Check sheet for the modelled part. Datum: model origin and axes. Units: mm. Face numbers are marked on the shaded views. A direction names the side the tool comes from. Round coordinates to 2 decimals unless told otherwise and drop trailing zeros. Write each loop counter-clockwise with the first axis right and the second up, starting at its lowest first coordinate (ties: lowest second). Pieces come first, ordered by that corner, then holes. Notation, with made-up numbers: M 60.25,-20 L 96.25,-20 A26 cw 96.25,9 Z; hole C 8,33 d2. An arc over 180 degrees is marked long. Answer in a Markdown table with one row per item.
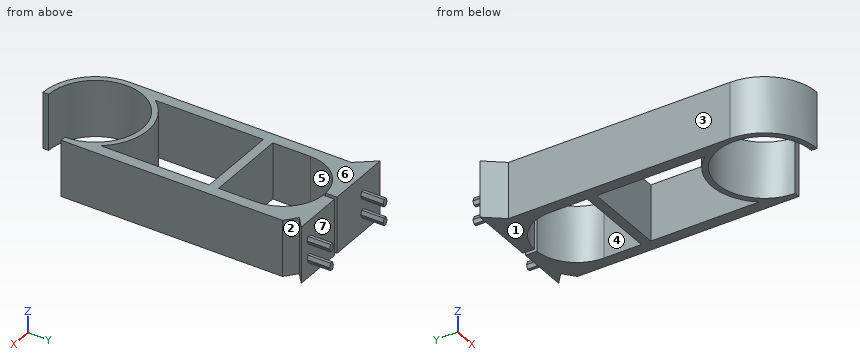
```python
from build123d import *

# Parameters (mm, degrees)
PAD_DEPTH    = 30
PAD001_DEPTH = 12


with BuildPart() as part:
    # Sketch → Pad (new body)
    with BuildSketch(Plane.XY):
        with BuildLine():
            ThreePointArc((25, 0), (-17.67767, 17.67767), (0, -25))
            Line((0, -25), (0, -28))
            ThreePointArc((-28, 1.4e-05), (-19.798995, -19.798985), (0, -28))
            Line((-28, 100.000014), (-28, 1.4e-05))
            Line((-28, 118.000014), (-28, 100.000014))
            Line((-36, 128), (-28, 118.000014))
            Line((-36, 128), (-1, 128))
            Line((-1, 128), (-1, 121.977261))
            ThreePointArc((-1, 121.977261), (-15.905969, 115.198689), (-22, 100.000014))
            Line((-22, 100.000014), (-22, 80))
            Line((-22, 80), (22, 80))
            Line((22, 100), (22, 80))
            ThreePointArc((22, 100), (15.905974, 115.198684), (1, 121.977261))
            Line((1, 128), (1, 121.977261))
            Line((1, 128), (28, 128))
            Line((28, 128), (22, 123))
            Line((22, 123), (28, 118))
            Line((28, 118), (28, 100))
            Line((28, 100), (28, 0))
            Line((25, 0), (28, 0))
        make_face()
        with BuildLine():
            ThreePointArc((22, 17.320508), (0, 28), (-22, 17.320508))
            Line((-22, 75), (-22, 17.320508))
            Line((-22, 75), (22, 75))
            Line((22, 75), (22, 17.320508))
        make_face(mode=Mode.SUBTRACT)
    extrude(amount=PAD_DEPTH)

    # Sketch001 (on Face13 of Pad) → Pad001 (join)
    with BuildSketch(Plane(origin=(0, 128, 0), x_dir=(-1, 0, 0), z_dir=(0, 1, 0))):
        Polygon((-22.5, 12), (-23.3, 10), (-22.5, 8), (-21, 8), (-20.2, 10), (-21, 12), align=None)
        Polygon((-22.5, 22), (-23.3, 20), (-22.5, 18), (-21, 18), (-20.2, 20), (-21, 22), align=None)
        Polygon((21, 12), (20.2, 10), (21, 8), (22.5, 8), (23.3, 10), (22.5, 12), align=None)
        Polygon((21, 22), (20.2, 20), (21, 18), (22.5, 18), (23.3, 20), (22.5, 22), align=None)
    extrude(amount=PAD001_DEPTH)


solid = part.part
```
1. Section check B-B, the plane z = 2.5. Record the cut outline in (x, y).
Found:
| item | result |
|---|---|
| outline | M -36,128 L -28,118 L -28,0 A28 ccw 0,-28 L 0,-25 A25 cw long 25,0 L 28,0 L 28,118 L 22,123 L 28,128 L 1,128 L 1,121.98 A22 cw 22,100 L 22,80 L -22,80 L -22,100 A22 cw -1,121.98 L -1,128 Z; hole M -22,17.32 A28 cw 22,17.32 L 22,75 L -22,75 Z |
2. Draft check along Y on the marked faces 5, 6 and 7. Enter one of: +Y half, -Y half, draft (parallel to the pull), parting line (faces both ways), or undercut.
Found:
| item | result |
|---|---|
| face 5 | undercut |
| face 6 | draft |
| face 7 | +Y half |
3. Section check D-D, the plane x = 13.5. Record the cut outline in (y, z), and give its area (3 significant figures).
Found:
| item | result |
|---|---|
| outline | M 21.04,0 L 24.53,0 L 24.53,30 L 21.04,30 Z; M 75,0 L 80,0 L 80,30 L 75,30 Z; M 117.37,0 L 128,0 L 128,30 L 117.37,30 Z |
| area | 574 mm2 |
4. Access from +Z, -Z, +X, -X, +Y, -Y to the whole of each face (thin tool, end or side, straight path). Record for the marked faces 1, 2, 3 and 4.
Found:
| item | result |
|---|---|
| face 1 | -Z, +X, -X, +Y, -Y |
| face 2 | +Z, -Z, +X |
| face 3 | +Z, -Z, -X, -Y |
| face 4 | +Z, -Z |
5. Scan lines: L1, parallel to X at y = 32.5, z = 24.25; L2, parallel to Y at x = 7, z = 9.5; L3, parallel to Y at x = -18.5, z = 8.25. Record each from-to range of solid material in increasing order.
Found:
| item | result |
|---|---|
| L1 | x = -28 to -22, 22 to 28 |
| L2 | y = 24 to 27.11, 75 to 80, 120.86 to 128 |
| L3 | y = -21.02 to -16.82, 16.82 to 21.02, 75 to 80, 111.91 to 128 |
6. Section check C-C, the plane x = -10. Record the cut outline in (y, z).
Found:
| item | result |
|---|---|
| outline | M -26.15,0 L -22.91,0 L -22.91,30 L -26.15,30 Z; M 22.91,0 L 26.15,0 L 26.15,30 L 22.91,30 Z; M 75,0 L 80,0 L 80,30 L 75,30 Z; M 119.6,0 L 128,0 L 128,30 L 119.6,30 Z |
7. Section check A-A, the plane y = 67. Record the cut outline in (x, z), and give its area (3 significant figures).
Found:
| item | result |
|---|---|
| outline | M -28,0 L -22,0 L -22,30 L -28,30 Z; M 22,0 L 28,0 L 28,30 L 22,30 Z |
| area | 360 mm2 |
8. Go/stop test with flat-tipped pins: pin 1 (1.6 mm diameter, centred on x = 22, y = 134, fed in from +Z); pin 2 (5 mm diameter, centred on x = -29, y = -11, fed in from +Z); pin 3 (1 mm diameter, centred on y = -0.5, z = 24.5, fed in from -X); pin 4 (10 mm diameter, centred on x = -6, z = 19.5, fed in from -Y). Record where each tip stops, or that it passes through.
Found:
| item | result |
|---|---|
| pin 1 | stops at z = 22 |
| pin 2 | passes through |
| pin 3 | stops at x = -28 |
| pin 4 | stops at y = -27.98 |
